from build123d import *

# Parameters (mm, degrees)
F1_DEPTH = 6.35
F3_DEPTH = 50.8
F4_R     = 10.515242
F5_DEPTH = 83.82


with BuildPart() as f1:
    # F0 (on Right) → F1 (new body)
    with BuildSketch(Plane.YZ):
        Polygon((41.387662, -35.488307), (41.387662, 46.365242), (18.896371, 46.365242), (-31.801209, -35.488307), align=None)
    extrude(amount=F1_DEPTH)

    # F2 (on face) → F3 (join)
    with BuildSketch(Plane(origin=(0, 0, 0), x_dir=(0, -1, 0), z_dir=(-1, 0, 0))):
        Polygon((-35.810284, -30.553309), (23.417182, -29.785352), (-20.715904, 41.469525), (-35.810284, 41.469525), align=None)
    extrude(amount=F3_DEPTH)

    # F4 (on face) → F5 (cut)
    with BuildSketch(Plane(origin=(0, -3.591343, 2.224368), x_dir=(1, 0, 0), z_dir=(0, -0.850143, 0.526552))):
        with Locations((-28.393257, 14.638352)):
            Circle(F4_R)
    extrude(amount=-F5_DEPTH, mode=Mode.SUBTRACT)


solid = f1.part
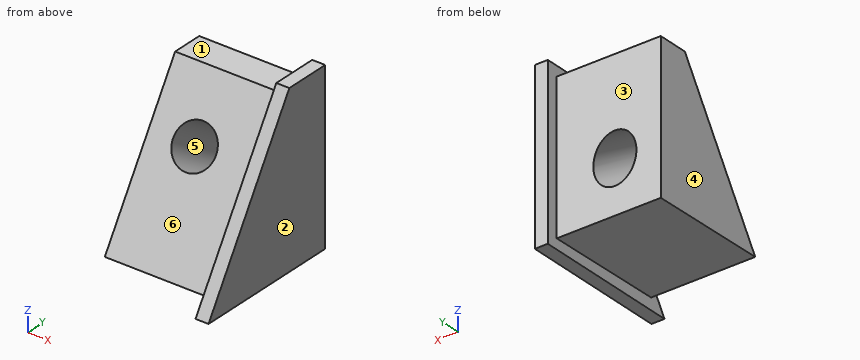
Check sheet for the modelled part. Datum: model origin and axes. Units: mm. Face numbers are marked on the shaded views. A direction names the side the tool comes from. Coordinates: 2 decimals unless noted, no trailing zeros. Write each loop counter-clockwise with the first axis right and the second up, starting at its lowest first coordinate (ties: lowest second). Pieces come first, ordered by that corner, then holes.
Item 1: Cross-section at D-D on x = -28.5. Record the boundary of the cut face in (y, z).
Numbers:
outline: (-23.42, -29.79) - (35.81, -30.55) - (35.81, -17.33) - (-1.42, 5.73) - close; (9.65, 23.61) - (35.81, 7.41) - (35.81, 41.47) - (20.72, 41.47) - close
Item 2: Cross-section at B-B on y = -8. Record the boundary of the cut face in (x, z).
Numbers:
outline: (-50.8, -29.99) - (0, -29.99) - (0, -35.49) - (6.35, -35.49) - (6.35, 2.94) - (0, 2.94) - (0, -4.89) - (-50.8, -4.89) - close
Item 3: Cross-section at A-A on x = -20.5. Record the boundary of the cut face in (y, z).
Numbers:
outline: (-23.42, -29.79) - (35.81, -30.55) - (35.81, -13.13) - (0.46, 8.76) - close; (7.77, 20.58) - (35.81, 3.21) - (35.81, 41.47) - (20.72, 41.47) - close
Item 4: Depth check by flat-ended pin: pin 1 Ø12 at (x, z) = (-41, -7.5) entering from +Y; pin 2 Ø2 at (x, z) = (-18.5, 30.5) entering from -Y; pin 3 Ø12 at (x, z) = (-21.5, 33.5) entering from -Y. Enter the tip coordinate at first touch or a pass-through.
Numbers:
pin 1: stops at y = 35.81
pin 2: stops at y = 13.3
pin 3: stops at y = 12.06
Item 5: Mould release check, pull along Z, two halves, no side actions. Record for the marked faces 4, 5 and 6: released by +Z, released by -Z, zero draft, split by the parting line, or undercut.
Numbers:
face 4: zero draft
face 5: undercut
face 6: released by +Z
Item 6: Access from +Z, -Z, +X, -X, +Y, -Y to the whole of each face (thin tool, end or side, straight path). Record for the marked faces 1, 2 and 3.
Numbers:
face 1: +Z, -X, +Y, -Y
face 2: +Z, -Z, +X, +Y, -Y
face 3: +Z, -Z, -X, +Y
Item 7: Scan lines: probe 1 along X at (y, z) = (9.5, 26); probe 2 along Z at (x, y) = (-29.5, 33.5); probe 3 along Z at (x, y) = (-31, 21). Record each from-to range of solid material in increasing order.
Numbers:
probe 1: x = 0 to 6.35
probe 2: z = -30.52 to -15.83, 8.77 to 41.47
probe 3: z = -30.36 to -7.77, 16.19 to 41.47
Item 8: Cross-section at C-C on x = -2.5. Record the boundary of the cut face in (y, z), then the cut area to 3 significant figures.
Numbers:
outline: (-23.42, -29.79) - (35.81, -30.55) - (35.81, 41.47) - (20.72, 41.47) - close
area: 2,670 mm2
